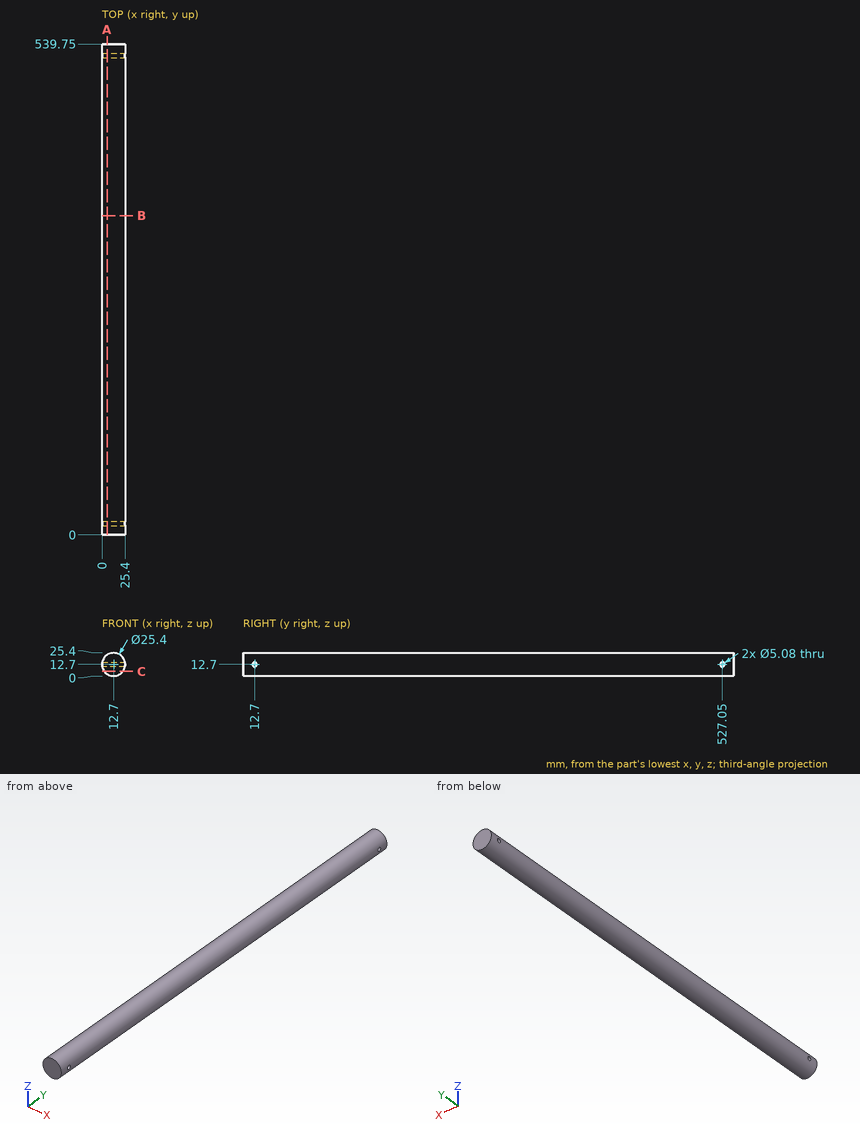
Design review of the part shown in the three views and the two pictorial views. Dimensions are in mm from the part's minimum x, y and z. Round coordinates to 2 decimals unless told otherwise and drop trailing zeros. Order: outer loops, then holes, each group sorted by start corner. A loop starts at its lowest first (then second) coordinate and runs counter-clockwise, first axis right, second up. Notation, with made-up numbers: (73.5, 37) - (112.5, 37) arc R30 ccw to (112.5, 72) - close; hole circle Ø5 at (-12, -26.5). An arc over 180 degrees is marked (long way). One line per question, with ' | ' between items.
Item 1: Take a section at A-A, the plane x = 5.5. Write out the cut boundary in (y, z).
Checks:
outline: (0, 2.24) - (539.75, 2.24) - (539.75, 23.16) - (0, 23.16) - close; hole circle Ø5.08 at (12.7, 12.7); hole circle Ø5.08 at (527.05, 12.7)
Item 2: Take a section at B-B, the plane y = 351. Write out the cut boundary in (x, z).
Checks:
outline: circle Ø25.4 at (12.7, 12.7)
Item 3: Wall thickness on line 1 (Y direction, x = 17.75, z = 12.7); line 2 (Y direction, x = 2, z = 13.75); line 3 (X direction, y = 316.5, z = 13.5): over which ranges is each line inside the solid? List them lowest first. Write a range as [from, to].
Checks:
line 1: [0, 10.16], [15.24, 524.51], [529.59, 539.75] | line 2: [0, 10.39], [15.01, 524.74], [529.36, 539.75] | line 3: [0.03, 25.37]
Item 4: For P1, Ø8, axis at x = 22, y = 164.5, coming from the +Z side; P2, Ø4, axis at x = 12, y = 451.5, coming from the -Z side; P3, Ø1, axis at y = 390, z = 19, coming from the +X side; P4, Ø2, axis at y = 231.5, z = 11, coming from the -X side, all flat-tipped, find the tip position at first contact; note any pin that passes through.
Checks:
P1: z = 24.24 | P2: z = 0 | P3: x = 24 | P4: x = 0.02
Item 5: Take a section at C-C, the plane z = 5. Write out the cut boundary in (x, y).
Checks:
outline: (2.6, 0) - (22.8, 0) - (22.8, 539.75) - (2.6, 539.75) - close
